from build123d import *

# Parameters (mm, degrees)
SKETCH_1_R      = 1.025
EXTRUDE_1_DEPTH = 25


with BuildPart() as part:
    # 草图1 → 凸台-拉伸1 (new body)
    with BuildSketch(Plane.XZ):
        Polygon((-1.443375673, -2.5), (1.443375673, -2.5), (2.886751346, 0), (1.443375673, 2.5), (-1.443375673, 2.5), (-2.886751346, 0), align=None)
        with Locations(Location((0, 0, 0), (0, 0, 90))):
            Circle(SKETCH_1_R, mode=Mode.SUBTRACT)
    extrude(amount=-EXTRUDE_1_DEPTH)


solid = part.part
Read the model definition and answer for the solid it produces. Units are mm, in the model's axes. Round coordinates to 2 decimals unless told otherwise and drop trailing zeros. Write each loop counter-clockwise with the first axis right and the second up, starting at its lowest first coordinate (ties: lowest second). Pieces come first, ordered by that corner, then holes.
Q1. A flat-ended cylindrical pin translates along its axis: P1, Ø1, axis at x = 2, y = 20.5, coming from the -Z side. Find the tip coordinate at first contact, or state that the pin passes through.
Values:
P1: stops at z = -2.4
Q2. The mould has two halves that part along X. Classify faces 1 (the face through (-2.155, 12.325, 1.267)), 2 (the face through (0, 12, -2.5)), 3 (the face through (2.175, 12.325, 1.233)), 4 (the face through (-1.016, 12.325, -0.133)): released by +X, released by -X, zero draft, split by the parting line, or undercut.
Values:
face 1: released by -X
face 2: zero draft
face 3: released by +X
face 4: undercut
Q3. Find section C-C on z = -0.5. Determine the outline of the cut face in (x, y).
Values:
outline: (-2.6, 0) - (-0.89, 0) - (-0.89, 25) - (-2.6, 25) - close; (0.89, 0) - (2.6, 0) - (2.6, 25) - (0.89, 25) - close
Q4. Find section D-D on z = 1.45. Determine the outline of the cut face in (x, y).
Values:
outline: (-2.05, 0) - (2.05, 0) - (2.05, 25) - (-2.05, 25) - close
Q5. Straight lines are drawn through the part: line 1 (Z direction, x = -0.8, y = 7.75); line 2 (Z direction, x = -0.15, y = 19.25); line 3 (X direction, y = 9.5, z = -0.6). For each, find the intervals that lie inside material, in ascending order.
Values:
line 1: z = -2.5 to -0.64, 0.64 to 2.5
line 2: z = -2.5 to -1.01, 1.01 to 2.5
line 3: x = -2.54 to -0.83, 0.83 to 2.54
Q6. Find section B-B on y = 15.5. Determine the outline of the cut face in (x, z) (3 decimals).
Values:
outline: (-2.887, 0) - (-1.443, -2.5) - (1.443, -2.5) - (2.887, 0) - (1.443, 2.5) - (-1.443, 2.5) - close; hole circle Ø2.05 at (0, 0)
Q7. Find section A-A on x = 0. Determine the outline of the cut face in (y, z) (3 decimals).
Values:
outline: (0, -2.5) - (25, -2.5) - (25, -1.025) - (0, -1.025) - close; (0, 1.025) - (25, 1.025) - (25, 2.5) - (0, 2.5) - close
